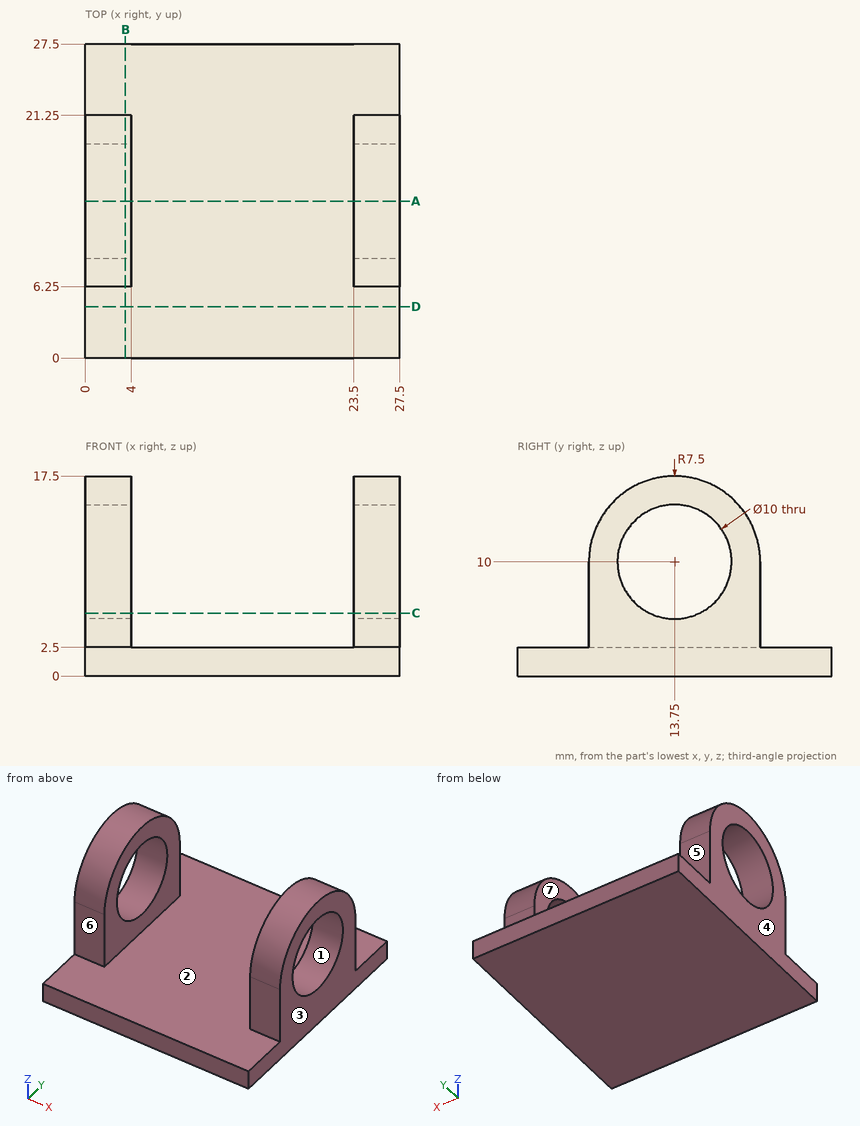
The drawing under review shows one solid part. Ordinate dimensions are in mm from its lowest x, y, z. A direction names the side the tool comes from. Round coordinates to 2 decimals unless told otherwise and drop trailing zeros. Write each loop counter-clockwise with the first axis right and the second up, starting at its lowest first coordinate (ties: lowest second). Pieces come first, ordered by that corner, then holes. Notation, with made-up numbers: (72.5, 55.5) - (129.5, 55.5) arc R15 ccw to (129.5, 78.5) - close; hole circle Ø7 at (66.25, 5). An arc over 180 degrees is marked (long way). Use a Markdown table: item, result. Add a question column.
1. We need section D-D (y = 4.5). State the section outline as (x, z) points, then the cut area to 4 significant figures.
2. We need section A-A (y = 13.75). State the section outline as (x, z) points.
3. Mouldability with a two-part tool opening along X and no side actions: class the marked faces 1, 2, 3 and 4 as +X half, -X half, draft (parallel to the pull), parting line (faces both ways), or undercut.
4. Clearance check with flat-ended pins moving along their axes: pin 1 (2 mm diameter, centred on x = 16.5, y = 23, fed in from +Z); pin 2 (4.5 mm diameter, centred on x = 1.5, z = 6.5, fed in from +Y); pin 3 (4 mm diameter, centred on x = 9, z = 2.5, fed in from -Y); pin 4 (2 mm diameter, centred on y = 14, z = 7.5, fed in from -X). State where each tip first meets the part, or that it passes through.
5. For the marked faces 5, 6 and 7, list the 3-axis set-ups (+Z, -Z, +X, -X, +Y, -Y) from which the entire face can be reached by the end or side of a thin tool; tool diameter is ignored.
6. We need section C-C (z = 5.5). State the section outline as (x, y) points, then the cut area to 3 significant figures.
7. We need section B-B (x = 3.5). State the section outline as (y, z) points, then the cut area to 3 significant figures.
8. Wall thickness on probe 1 along X at (y, z) = (9.75, 13.5); probe 2 along Y at (x, z) = (26.5, 10); probe 3 along Z at (x, y) = (8.25, 2.5): over which ranges is each line inside the solid? List them lowest first.
Output:
| question | item | result |
|---|---|---|
| 1 | outline | (0, 0) - (27.5, 0) - (27.5, 2.5) - (0, 2.5) - close |
| 1 | area | 68.75 mm2 |
| 2 | outline | (0, 0) - (27.5, 0) - (27.5, 5) - (23.5, 5) - (23.5, 2.5) - (4, 2.5) - (4, 5) - (0, 5) - close; (0, 15) - (4, 15) - (4, 17.5) - (0, 17.5) - close; (23.5, 15) - (27.5, 15) - (27.5, 17.5) - (23.5, 17.5) - close |
| 3 | face 1 | draft |
| 3 | face 2 | undercut |
| 3 | face 3 | +X half |
| 3 | face 4 | -X half |
| 4 | pin 1 | stops at z = 2.5 |
| 4 | pin 2 | stops at y = 21.25 |
| 4 | pin 3 | stops at y = 0 |
| 4 | pin 4 | passes through |
| 5 | face 5 | +Z, +X, -X, +Y |
| 5 | face 6 | +Z, +X, -X, -Y |
| 5 | face 7 | +Z, +Y, -Y |
| 6 | outline | (0, 6.25) - (4, 6.25) - (4, 11.57) - (0, 11.57) - close; (0, 15.93) - (4, 15.93) - (4, 21.25) - (0, 21.25) - close; (23.5, 6.25) - (27.5, 6.25) - (27.5, 11.57) - (23.5, 11.57) - close; (23.5, 15.93) - (27.5, 15.93) - (27.5, 21.25) - (23.5, 21.25) - close |
| 6 | area | 85.1 mm2 |
| 7 | outline | (0, 0) - (27.5, 0) - (27.5, 2.5) - (21.25, 2.5) - (21.25, 10) arc R7.5 ccw to (6.25, 10) - (6.25, 2.5) - (0, 2.5) - close; hole circle Ø10 at (13.75, 10) |
| 7 | area | 191 mm2 |
| 8 | probe 1 | x = 0 to 4, 23.5 to 27.5 |
| 8 | probe 2 | y = 6.25 to 8.75, 18.75 to 21.25 |
| 8 | probe 3 | z = 0 to 2.5 |
